```python
from build123d import *

# Parameters (mm, degrees)
F0_W      = 115
F0_H      = 75
F1_DEPTH  = 25
F2_DEPTH  = 75
F4_DEPTH  = 75.001
F6_DEPTH  = 50
F7_W      = 55
F7_H      = 25
F8_DEPTH  = 50.001
F9_W      = 35
F9_H      = 49
F10_DEPTH = 25.001
F11_W     = 30
F11_H     = 10
F12_DEPTH = 15
F13_W     = 30
F13_H     = 10
F14_DEPTH = 15


with BuildPart() as f1:
    # F0 (on Top) → F1 (new body)
    with BuildSketch(Plane.XY):
        with Locations((2.0555268228, -8.5665475577)):
            Rectangle(F0_W, F0_H)
    extrude(amount=F1_DEPTH)

    # F0 (on Top) → F2 (join)
    with BuildSketch(Plane.XY):
        with Locations((2.0555268228, -8.5665475577)):
            Rectangle(F0_W, F0_H)
    extrude(amount=F2_DEPTH)

    # F3 (on face) → F4 (cut, through all)
    with BuildSketch(Plane.XZ.offset(46.0665475577)):
        Polygon((-40.4444731772, 12), (-40.4444731772, 0), (-1.3980267197, 0), (44.5555268228, 0), (44.5555268228, 12), align=None)
    extrude(amount=-F4_DEPTH, mode=Mode.SUBTRACT)

    # F5 (on face) → F6 (cut)
    with BuildSketch(Plane.XY.offset(75)):
        Polygon((59.5555268228, 28.9334524423), (-5.4444731772, 28.9334524423), (-5.4444731772, 18.9334524423), (-5.4444731772, -36.0665475577), (-5.4444731772, -46.0665475577), (59.5555268228, -46.0665475577), align=None)
    extrude(amount=-F6_DEPTH, mode=Mode.SUBTRACT)

    # F7 (on face) → F8 (cut, through all)
    with BuildSketch(Plane.YZ.offset(-5.4444731772)):
        with Locations((-8.5665475577, 62.5)):
            Rectangle(F7_W, F7_H)
    extrude(amount=-F8_DEPTH, mode=Mode.SUBTRACT)

    # F9 (on face) → F10 (cut, through all)
    with BuildSketch(Plane.XY.offset(25)):
        with Locations((27.0555268228, -8.5665475577)):
            Rectangle(F9_W, F9_H)
    extrude(amount=-F10_DEPTH, mode=Mode.SUBTRACT)

    # F11 (on face) → F12 (cut)
    with BuildSketch(Plane.XY.offset(75)):
        with Locations((-30.4444731772, 23.9334524423)):
            Rectangle(F11_W, F11_H)
    extrude(amount=-F12_DEPTH, mode=Mode.SUBTRACT)

    # F13 (on face) → F14 (cut)
    with BuildSketch(Plane.XY.offset(75)):
        with Locations((-30.4444731772, -41.0665475577)):
            Rectangle(F13_W, F13_H)
    extrude(amount=-F14_DEPTH, mode=Mode.SUBTRACT)


solid = f1.part
```
Check sheet for the modelled part. Datum: model origin and axes. Units: mm. A direction names the side the tool comes from. Coordinates: 2 decimals unless noted, no trailing zeros. Write each loop counter-clockwise with the first axis right and the second up, starting at its lowest first coordinate (ties: lowest second). Pieces come first, ordered by that corner, then holes. Notation, with made-up numbers: (63.5, -2) - (72.5, -2) arc R7 ccw to (72.5, 3) - close; hole circle Ø4 at (-9, -31). An arc over 180 degrees is marked (long way). One line per question, with ' | ' between items.
Item 1: Sectioned sample at A-A on z = 57.5. Record the boundary of the cut face in (x, y), plus the area to 3 significant figures.
Determined:
outline: (-55.44, -46.07) - (-5.44, -46.07) - (-5.44, -36.07) - (-55.44, -36.07) - close; (-55.44, 18.93) - (-5.44, 18.93) - (-5.44, 28.93) - (-55.44, 28.93) - close | area: 1,000 mm2
Item 2: Mould release check, pull along Y, two halves, no side actions. Record for faces 5 (the face through (27, 15.933, 19)), 6 (the face through (9.556, -9, 19)), 7 (the face through (59.556, -9, 12)): pulls with the +Y half, pulls with the -Y half, needs draft (parallel to the pull), parting line crosses it, or undercut.
Determined:
face 5: undercut | face 6: undercut | face 7: needs draft
Item 3: Sectioned sample at B-B on x = 14. Record the boundary of the cut face in (y, z).
Determined:
outline: (-46.07, 12) - (-33.07, 12) - (-33.07, 25) - (-46.07, 25) - close; (15.93, 12) - (28.93, 12) - (28.93, 25) - (15.93, 25) - close
Item 4: Gauge pin test, flat ends, axial feed: P1, Ø5, axis at x = -26.5, y = 22, coming from the +Z side; P2, Ø10, axis at x = -43, y = 13.5, coming from the -Z side; P3, Ø5, axis at y = 23.5, z = 68.5, coming from the +X side; P4, Ø15, axis at x = -34, y = -22, coming from the +Z side. Record the tip position at first contact, or that the pin passes through.
Determined:
P1: stops at z = 60 | P2: stops at z = 0 | P3: stops at x = -5.44 | P4: stops at z = 50
Item 5: Thickness scan on line 1 (X direction, y = 10.5, z = 19.5); line 2 (X direction, y = -42, z = 70); line 3 (Y direction, x = -21.5, z = 53.5). Record the ranges inside material, lowest first. Write a range as [from, to].
Determined:
line 1: x = [-55.44, 9.56], [44.56, 59.56] | line 2: x = [-55.44, -45.44], [-15.44, -5.44] | line 3: y = [-46.07, -36.07], [18.93, 28.93]
Item 6: Sectioned sample at C-C on z = 65. Record the boundary of the cut face in (x, y), plus the area to 3 significant figures.
Determined:
outline: (-55.44, -46.07) - (-45.44, -46.07) - (-45.44, -36.07) - (-55.44, -36.07) - close; (-55.44, 18.93) - (-45.44, 18.93) - (-45.44, 28.93) - (-55.44, 28.93) - close; (-15.44, -46.07) - (-5.44, -46.07) - (-5.44, -36.07) - (-15.44, -36.07) - close; (-15.44, 18.93) - (-5.44, 18.93) - (-5.44, 28.93) - (-15.44, 28.93) - close | area: 400 mm2
Item 7: Sectioned sample at D-D on y = -10. Record the boundary of the cut face in (x, z).
Determined:
outline: (-55.44, 0) - (-40.44, 0) - (-40.44, 12) - (9.56, 12) - (9.56, 25) - (-5.44, 25) - (-5.44, 50) - (-55.44, 50) - close; (44.56, 0) - (59.56, 0) - (59.56, 25) - (44.56, 25) - close
Item 8: Access from +Z, -Z, +X, -X, +Y, -Y to the whole of each face (thin tool, end or side, straight path). Record for faces 1 (the face through (-40.444, -9, 6)), 2 (the face through (-31, 24, 60)), 3 (the face through (48, -8, 25)), 4 (the face through (27, -33.067, 19)).
Determined:
face 1: -Z, +Y, -Y | face 2: +Z, +Y, -Y | face 3: +Z, +X, +Y, -Y | face 4: +Z, -Z
